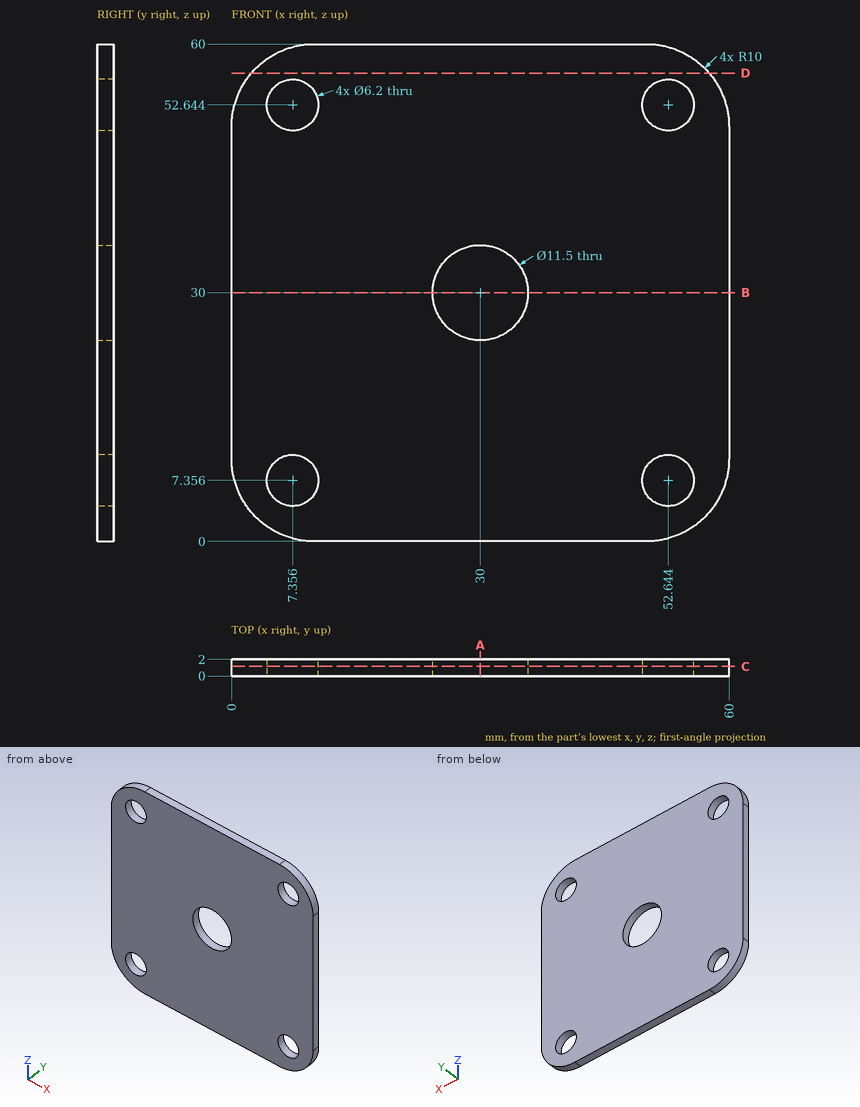
Verification items for this drawing (mm, ordinates from the low corner). Round coordinates to 2 decimals unless told otherwise and drop trailing zeros. Order: outer loops, then holes, each group sorted by start corner. A loop starts at its lowest first (then second) coordinate and runs counter-clockwise, first axis right, second up. Notation, with made-up numbers: (-10.75, 49) - (9.25, 49) arc R17 cw to (9.25, 62) - close; hole circle Ø1 at (76.25, -15). An arc over 180 degrees is marked (long way). Answer as CSV lines item,"result". Start each with the question number.
1) Scan lines: probe 1 along Z at (x, y) = (54, 1) (1 decimal); probe 2 along Z at (x, y) = (6.5, 1.45) (1 decimal); probe 3 along Z at (x, y) = (30, 0.9). Record each from-to range of solid material in increasing order.
2) Section check D-D (z = 56.5). Record the cut outline in (x, y).
3) Section check C-C (y = 1.15). Record the cut outline in (x, z).
4) Section check A-A (x = 30). Record the cut outline in (y, z), then the cut area to 3 significant figures.
5) Section check B-B (z = 30). Record the cut outline in (x, y), then the cut area to 3 significant figures.
Determined:
1,probe 1,"0.8 to 4.6, 10.1 to 49.9, 55.4 to 59.2"
1,probe 2,"0.6 to 4.4, 10.3 to 49.7, 55.6 to 59.4"
1,probe 3,"0 to 24.25, 35.75 to 60"
2,outline,"(2.4, 0) - (57.6, 0) - (57.6, 2) - (2.4, 2) - close"
3,outline,"(0, 10) arc R10 ccw to (10, 0) - (50, 0) arc R10 ccw to (60, 10) - (60, 50) arc R10 ccw to (50, 60) - (10, 60) arc R10 ccw to (0, 50) - close; hole circle Ø6.2 at (7.36, 7.36); hole circle Ø6.2 at (7.36, 52.64); hole circle Ø11.5 at (30, 30); hole circle Ø6.2 at (52.64, 7.36); hole circle Ø6.2 at (52.64, 52.64)"
4,outline,"(0, 0) - (2, 0) - (2, 24.25) - (0, 24.25) - close; (0, 35.75) - (2, 35.75) - (2, 60) - (0, 60) - close"
4,area,"97.0 mm^2"
5,outline,"(0, 0) - (24.25, 0) - (24.25, 2) - (0, 2) - close; (35.75, 0) - (60, 0) - (60, 2) - (35.75, 2) - close"
5,area,"97.0 mm^2"
